Can you work these out from the model? Positions are in its coordinate system, mm. Give positions to 0.01 mm unless a question says otherwise; leave off trailing zeros. Write each loop counter-clockwise with the first axis right and the second up, starting at its lowest first coordinate (ties: lowest second). Pieces come first, ordered by that corner, then holes.
1. I'm going to push flat-ended pins straight in: pin 1 (3 mm diameter, centred on x = 63.5, y = 11, fed in from +Z); pin 2 (7.5 mm diameter, centred on x = -63.5, y = 11, fed in from +Z). Where does each tip first touch, or does it pass through?
2. If I drill on probe 1 along X at (y, z) = (1, 1.7); probe 2 along Y at (x, z) = (-18.5, 2.4); probe 3 along X at (y, z) = (12.25, 3.05), over which ranges is the centre line in solid material (lowest first)?
3. Suppose I cut it at A-A (y = 11). Give the number of separate pieces and of enclosed holes in the cut face, and give its area (3 significant figures).
4. Suppose I cut it at B-B (y = 1). Please give me the cut outline in (x, z).
5. Suppose I cut it at D-D (z = 2.15). Please give me the cut outline in (x, y), and give its area (3 significant figures).
6. Thinking about a two-plate mould opening in Y: for faces 1 (the flat face through (1, 20, 2)), 2 (the flat face through (72.5, 6, 2)), 3 (the cylindrical face through (16.157, 11.52, 1.572)), which applies, pulls with the +Y half, pulls with the -Y half, needs draft (parallel to the pull), parting line crosses it, or undercut?
7. Suppose I cut it at C-C (x = 63.5). Please give me the cut outline in (y, z).
Solid Edge part; units mm, degrees
sketch "Sketch1" plane through (0, 0, 0) normal (0, 0, 1) x (1, 0, 0)
  line L0 (-72.5, -20) -> (72.5, -20)
  line L1 (72.5, -20) -> (72.5, 20)
  line L2 (72.5, 20) -> (-72.5, 20)
  line L3 (-72.5, 20) -> (-72.5, -20)
extrude "Protrusion1" add sketch "Sketch1" along normal blind 5
hole "Bohrung_1" at (-63.5, 11, 5) direction (0, 0, -1) diameter 4.8 end up to next countersink diameter 8.6 countersink angle 90
hole "Hole1" at (-18.5, 11, 5) direction (0, 0, -1) diameter 4.8 end up to next countersink diameter 8.6 countersink angle 90
hole "Hole2" at (18.5, 11, 5) direction (0, 0, -1) diameter 4.8 end up to next countersink diameter 8.6 countersink angle 90
hole "Hole3" at (63.5, 11, 5) direction (0, 0, -1) diameter 4.8 end up to next countersink diameter 8.6 countersink angle 90
hole "Hole4" at (41, 1, 5) direction (0, 0, -1) diameter 4.8 end up to next countersink diameter 8.6 countersink angle 90
hole "Hole5" at (0, 1, 5) direction (0, 0, -1) diameter 4.8 end up to next countersink diameter 8.6 countersink angle 90
hole "Hole6" at (-41, 1, 5) direction (0, 0, -1) diameter 4.8 end up to next countersink diameter 8.6 countersink angle 90
sketch "Sketch2" plane through (-72.5, 0, 2.5) normal (-1, 0, 0) x (0, 1, 0)
  line L0 (-7.5, 2.5) -> (-7.5, -2.5)
  line L1 (-7.5, -2.5) -> (-21.6634, -3.36)
  line L2 (-21.6634, -3.36) -> (-22.4966, 5.1713)
  line L3 (-22.4966, 5.1713) -> (-7.5, 2.5)
extrude "Extrusionsausschnitt_1" cut sketch "Sketch2" against normal blind 163.0686
fillet "Verrundung_1" radius 1 4 edges at (-72.5, 6.25, 5) (0, 20, 5) (72.5, 6.25, 5) (0, -7.5, 5)
fillet "Verrundung_2" radius 3 8 edges at (-72.5, 20, 2) (-72.2071, 19.7071, 4.7071) (-72.2071, -7.2071, 4.7071) (-72.5, -7.5, 2) (72.5, 20, 2) (72.2071, 19.7071, 4.7071) (72.5, -7.5, 2) (72.2071, -7.2071, 4.7071)
fillet "Verrundung_3" radius 1 7 edges at (-72.5, 6.25, 0) (-71.6213, -6.6213, 0) (0, -7.5, 0) (71.6213, -6.6213, 0) (72.5, 6.25, 0) (0, 20, 0) (-71.6213, 19.1213, 0)
Checks:
1. pin 1: passes through
1. pin 2: stops at z = 4.45
2. probe 1: x = -72.5 to -43.4, -38.6 to -2.4, 2.4 to 38.6, 43.4 to 72.5
2. probe 2: y = -7.5 to 8.6, 13.4 to 20
2. probe 3: x = -72.5 to -65.55, -61.45 to -20.55, -16.45 to 16.45, 20.55 to 61.45, 65.55 to 72.5
3. separate pieces: 5
3. enclosed holes: 0
3. area: 614 mm2
4. outline: (-72.5, 1) arc R1 ccw to (-71.5, 0) - (-43.4, 0) - (-43.4, 3.1) - (-45.3, 5) - (-71.5, 5) arc R1 ccw to (-72.5, 4) - close; (-38.6, 0) - (-2.4, 0) - (-2.4, 3.1) - (-4.3, 5) - (-36.7, 5) - (-38.6, 3.1) - close; (2.4, 0) - (38.6, 0) - (38.6, 3.1) - (36.7, 5) - (4.3, 5) - (2.4, 3.1) - close; (43.4, 0) - (71.5, 0) arc R1 ccw to (72.5, 1) - (72.5, 4) arc R1 ccw to (71.5, 5) - (45.3, 5) - (43.4, 3.1) - close
5. outline: (-72.5, -4.5) arc R3 ccw to (-69.5, -7.5) - (69.5, -7.5) arc R3 ccw to (72.5, -4.5) - (72.5, 17) arc R3 ccw to (69.5, 20) - (-69.5, 20) arc R3 ccw to (-72.5, 17) - close; hole circle Ø4.8 at (-63.5, 11); hole circle Ø4.8 at (-41, 1); hole circle Ø4.8 at (-18.5, 11); hole circle Ø4.8 at (0, 1); hole circle Ø4.8 at (18.5, 11); hole circle Ø4.8 at (41, 1); hole circle Ø4.8 at (63.5, 11)
5. area: 3,850 mm2
6. face 1: pulls with the +Y half
6. face 2: needs draft
6. face 3: undercut
7. outline: (-7.5, 1) arc R1 ccw to (-6.5, 0) - (8.6, 0) - (8.6, 3.1) - (6.7, 5) - (-6.5, 5) arc R1 ccw to (-7.5, 4) - close; (13.4, 0) - (19, 0) arc R1 ccw to (20, 1) - (20, 4) arc R1 ccw to (19, 5) - (15.3, 5) - (13.4, 3.1) - close
